Geometry: see drawing. Coordinates: mm, zero at the bounding-box minimum. Round coordinates to 2 decimals unless told otherwise and drop trailing zeros. Order: outer loops, then holes, each group sorted by start corner. A loop starts at its lowest first (then second) coordinate and runs counter-clockwise, first axis right, second up. Notation, with made-up numbers: (-31, -23) -> (-17, -23) arc R29 cw to (-17, -3) -> close; hole circle Ø9 at (-11, 58.5). An arc over 180 degrees is marked (long way). Answer as CSV lines item,"result". Start each with the question number.
(1) Pull-direction query (Y, two-part tool) for the marked faces 1, 2 and 3; classes: +Y half, -Y half, draft (parallel to the pull), parting line (faces both ways), or undercut.
(2) Section query D-D (x = 31). Output: boundary loops of the cut face in (y, z).
(3) Contact query for flat-ended pins moving along their axis: P1, Ø3, axis at x = 25, z = 39.5, coming from the -Y side; P2, Ø8, axis at y = 37.5, z = 72, coming from the +X side (3 decimals); P3, Ø8, axis at y = 9.5, z = 33, coming from the -X side. Output: stop coordinate, or through.
(4) Section query A-A (x = 22). Output: boundary loops of the cut face in (y, z).
(5) Line query: line 1 along Y through (x, z) = (22, 8); line 2 along Z through (x, y) = (38, 23.5); line 3 along Y through (x, z) = (22, 86). Output: solid intervals per line, ascending. Write a range as from..to.
(6) Section query C-C (z = 32.5). Output: boundary loops of the cut face in (x, y), plus the area to 3 significant figures.
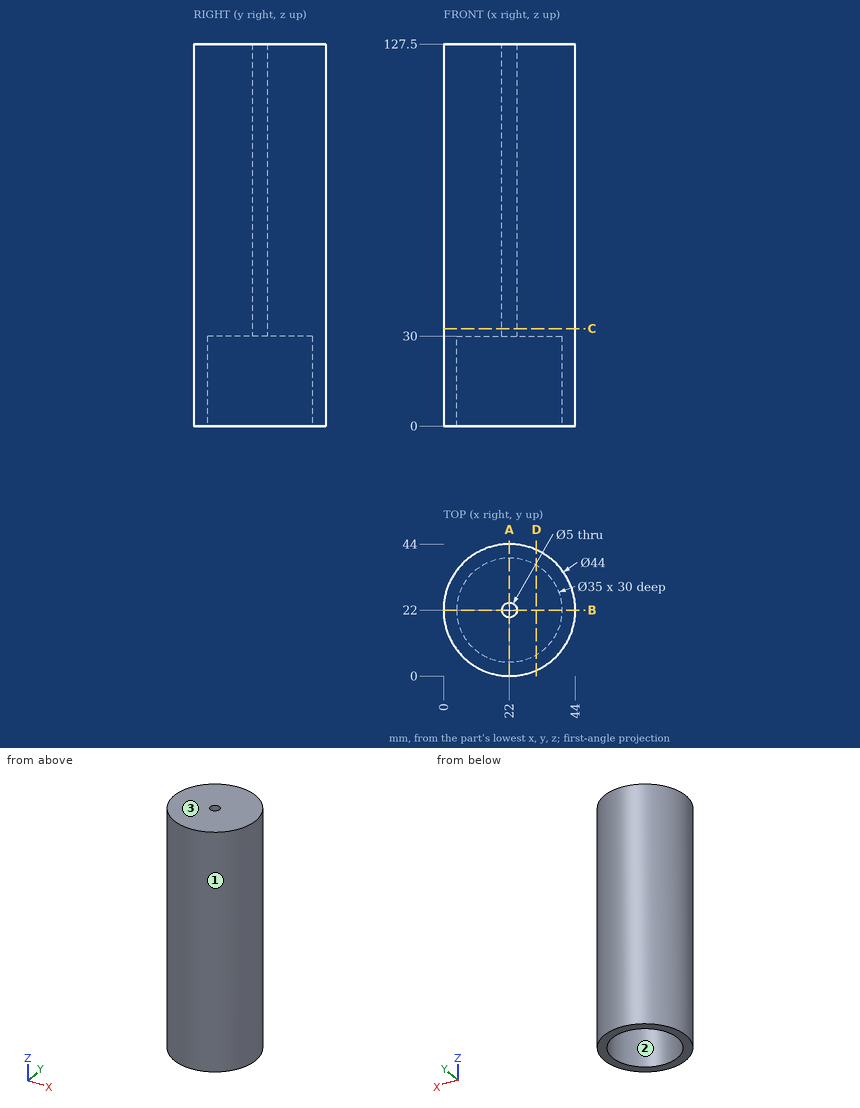
Answer block:
1,face 1,"parting line"
1,face 2,"undercut"
1,face 3,"draft"
2,outline,"(1.93, 0) -> (6.99, 0) -> (6.99, 30) -> (37.01, 30) -> (37.01, 0) -> (42.07, 0) -> (42.07, 127.5) -> (1.93, 127.5) -> close"
3,P1,"y = 0.05"
3,P2,"x = 40.755"
3,P3,"x = 1.71"
4,outline,"(0, 0) -> (4.5, 0) -> (4.5, 30) -> (19.5, 30) -> (19.5, 127.5) -> (0, 127.5) -> close; (24.5, 30) -> (39.5, 30) -> (39.5, 0) -> (44, 0) -> (44, 127.5) -> (24.5, 127.5) -> close"
5,line 1,"0..4.5, 39.5..44"
5,line 2,"30..127.5"
5,line 3,"0..19.5, 24.5..44"
6,outline,"circle Ø44 at (22, 22); hole circle Ø5 at (22, 22)"
6,area,"1,500 mm2"
